```python
from build123d import *

# Parameters (mm, degrees)
F0_R     = 16
F1_DEPTH = 47.5
F3_DEPTH = 95
F5_D     = 15


# Not quite as in the source:
# - ends of sketch curves that miss each other by under 0.0002 mm in the source are joined


with BuildPart() as f1:
    # F0 (on Top) → F1 (new body, symmetric)
    with BuildSketch(Plane.XY):
        Polygon((95, 0), (0, 0), (-95, 0), (-67.5, -55), (-95, -125), (0, -125), (95, -125), (67.5, -55), align=None)
        with Locations((0, -70)):
            Circle(F0_R, mode=Mode.SUBTRACT)
    extrude(amount=F1_DEPTH, both=True)

    # F2 (on Right) → F3 (intersect, symmetric)
    with BuildSketch(Plane.YZ):
        with BuildLine():
            Line((-10, 0), (0, 0))
            Line((0, 0), (0, 37.5))
            ThreePointArc((0, 37.5), (-2.9289321881, 44.5710678119), (-10, 47.5))
            Line((-10, 47.5), (-53, 47.5))
            ThreePointArc((-53, 47.5), (-54.4142135624, 46.9142135624), (-55, 45.5))
            Line((-55, 45.5), (-55, 41.5))
            ThreePointArc((-55, 41.5), (-56.1715728753, 38.6715728753), (-59, 37.5))
            Line((-59, 37.5), (-103, 37.5))
            ThreePointArc((-103, 37.5), (-112.8615414617, 40.1853795152), (-120, 47.5))
            Line((-120, 47.5), (-124.3701794471, 45.0706943661))
            ThreePointArc((-124.3701794471, 45.0706943661), (-115.3966418036, 35.8757089339), (-103, 32.5000005737))
            Line((-103, 32.5000005737), (-50, 32.5000005737))
            ThreePointArc((-50, 32.5000005737), (-48.5355339059, 36.0355339059), (-45, 37.5))
            Line((-45, 37.5), (-10, 37.5))
            Line((-10, 37.5), (-10, 0))
        make_face()
        with BuildLine():
            Line((0, -37.5), (0, 0))
            Line((0, 0), (-10, 0))
            Line((-10, 0), (-10, -37.5))
            Line((-10, -37.5), (-45, -37.5))
            ThreePointArc((-45, -37.5), (-48.5355339059, -36.0355339059), (-50, -32.5))
            Line((-50, -32.5), (-103, -32.5000005737))
            ThreePointArc((-103, -32.5000005737), (-115.3966418036, -35.8757089339), (-124.3701794471, -45.0706943661))
            Line((-124.3701794471, -45.0706943661), (-120, -47.5))
            ThreePointArc((-120, -47.5), (-112.8615414617, -40.1853795152), (-103, -37.5))
            Line((-103, -37.5), (-59, -37.5))
            ThreePointArc((-59, -37.5), (-56.1715728753, -38.6715728753), (-55, -41.5))
            Line((-55, -41.5), (-55, -45.5))
            ThreePointArc((-55, -45.5), (-54.4142135624, -46.9142135624), (-53, -47.5))
            Line((-53, -47.5), (-10, -47.5))
            ThreePointArc((-10, -47.5), (-2.9289321881, -44.5710678119), (0, -37.5))
        make_face()
    extrude(amount=F3_DEPTH, both=True, mode=Mode.INTERSECT)

    # F5 (through all)
    with Locations(Plane(origin=(0, 0, 0), x_dir=(-1, 0, 0), z_dir=(0, 1, 0))):
        with Locations((67.5, 0), (-67.5, 0)):
            Hole(F5_D / 2)


solid = f1.part
```
Here's how the part is built. I have some questions about the finished solid (model axes, mm). A direction names the side the tool comes from. Coordinates: 2 decimals unless noted, no trailing zeros. Order: outer loops, then holes, each group sorted by start corner. A loop starts at its lowest first (then second) coordinate and runs counter-clockwise, first axis right, second up.
1) Imagine slicing it at A-A on y = -29.5. List the corners of the cut face in (x, z) for me, and give its area (3 significant figures).
2) Will these pins go through, and if not, where does the flat tip stop? pin 1 (5 mm diameter, centred on x = -62, z = -16.5, fed in from -Y); pin 2 (1.2 mm diameter, centred on x = -33.5, z = 44, fed in from -Y); pin 3 (1.2 mm diameter, centred on x = -49.5, z = -43.5, fed in from -Y); pin 4 (12 mm diameter, centred on y = -20.5, z = -22.5, fed in from -X).
3) We'd pull the mould along X, two halves only. Please class faces 4 (the face through (1, 0, -1)), 5 (the face through (81.19, -89.85, 35.59)), 6 (the face through (-75, -5, 0)), 7 (the face through (-2.083, -54.136, -36.698)): +X half, -X half, draft (parallel to the pull), parting line (faces both ways), or undercut.
4) Imagine slicing it at B-B on x = 0. List the corners of the cut face in (y, z) for me.
5) Imagine slicing it at D-D on y = -67. List the corners of the cut face in (x, z) for me, and give its area (3 significant figures).
6) Imagine slicing it at C-C on z = 0. List the corners of the cut face in (x, y) for me, and give its area (3 significant figures).
7) Which directions (+Z, -Z, +X, -X, +Y, -Y) give clear straight access to the entire face, cutting with the end or side of a thin tool? Please do faces 1 (the face through (37, -55, -43)), 2 (the face through (1, -28, 37.5)), 3 (the face through (1.327, -115.239, -35.784)).
8) I need wall thicknesses on line 1 (Z direction, x = 35.5, y = -23.5); line 2 (Z direction, x = 24.5, y = -95.5); line 3 (Y direction, x = 59.5, z = -34.5). Which ranges of each line are inside material? Lowest first, please.
Response values:
1. outline: (-80.25, -47.5) - (80.25, -47.5) - (80.25, -37.5) - (-80.25, -37.5) - close; (-80.25, 37.5) - (80.25, 37.5) - (80.25, 47.5) - (-80.25, 47.5) - close
1. area: 3,210 mm2
2. pin 1: stops at y = -10
2. pin 2: stops at y = -124.1
2. pin 3: stops at y = -123.8
2. pin 4: passes through
3. face 4: draft
3. face 5: +X half
3. face 6: undercut
3. face 7: undercut
4. outline: (-124.37, -45.07) - (-120, -47.5) arc R19.45 cw to (-103, -37.5) - (-86, -37.5) - (-86, -32.5) - (-103, -32.5) arc R24.45 ccw to start; (-124.37, 45.07) arc R24.45 ccw to (-103, 32.5) - (-86, 32.5) - (-86, 37.5) - (-103, 37.5) arc R19.45 cw to (-120, 47.5) - close; (-54, -47.23) arc R2 ccw to (-53, -47.5) - (-10, -47.5) arc R10 ccw to (0, -37.5) - (0, 37.5) arc R10 ccw to (-10, 47.5) - (-53, 47.5) arc R2 ccw to (-54, 47.23) - (-54, 32.5) - (-50, 32.5) arc R5 cw to (-45, 37.5) - (-10, 37.5) - (-10, -37.5) - (-45, -37.5) arc R5 cw to (-50, -32.5) - (-54, -32.5) - close
5. outline: (-72.21, -37.5) - (-15.72, -37.5) - (-15.72, -32.5) - (-72.21, -32.5) - close; (-72.21, 32.5) - (-15.72, 32.5) - (-15.72, 37.5) - (-72.21, 37.5) - close; (15.72, -37.5) - (72.21, -37.5) - (72.21, -32.5) - (15.72, -32.5) - close; (15.72, 32.5) - (72.21, 32.5) - (72.21, 37.5) - (15.72, 37.5) - close
5. area: 1,130 mm2
6. outline: (-95, 0) - (-90, -10) - (-75, -10) - (-75, 0) - close; (-60, -10) - (60, -10) - (60, 0) - (-60, 0) - close; (75, -10) - (90, -10) - (95, 0) - (75, 0) - close
6. area: 1,550 mm2
7. face 1: -Z, +X, -X
7. face 2: +X, -X
7. face 3: +X, -X, -Y
8. line 1: z = -47.5 to -37.5, 37.5 to 47.5
8. line 2: z = -37.5 to -32.5, 32.5 to 37.5
8. line 3: y = -112.69 to -49.58, -10 to 0
